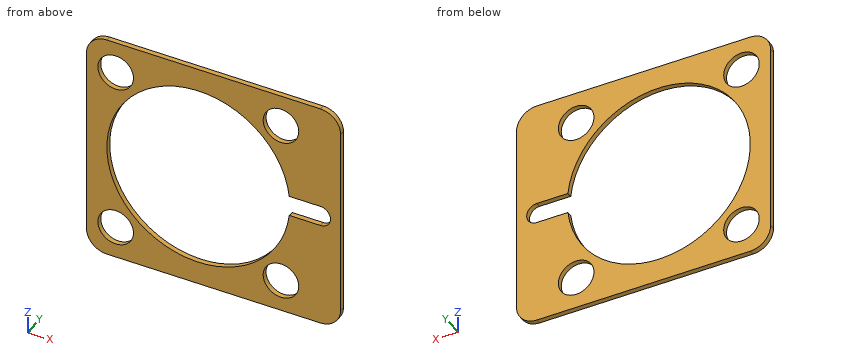
from build123d import *

# Parameters (mm, degrees)
SKETCH1_R           = 3.5
BOSS_EXTRUDE1_DEPTH = 1


with BuildPart() as part:
    # Sketch1 → Boss-Extrude1 (new body)
    with BuildSketch(Plane(origin=(0, 0, 0), x_dir=(1, 0, 0), z_dir=(0, 1, 0))):
        with BuildLine():
            Line((-21, -22.5), (21, -22.5))
            ThreePointArc((21, -22.5), (23.828427125, -21.328427125), (25, -18.5))
            Line((25, -18.5), (25, 18.5))
            ThreePointArc((25, 18.5), (23.828427125, 21.328427125), (21, 22.5))
            Line((21, 22.5), (-21, 22.5))
            ThreePointArc((-21, 22.5), (-23.828427125, 21.328427125), (-25, 18.5))
            Line((-25, 18.5), (-25, -18.5))
            ThreePointArc((-25, -18.5), (-23.828427125, -21.328427125), (-21, -22.5))
        make_face()
        with Locations((-19.263455967, 16.263455967)):
            Circle(SKETCH1_R, mode=Mode.SUBTRACT)
        with Locations((13.263455967, 16.263455967)):
            Circle(SKETCH1_R, mode=Mode.SUBTRACT)
        with Locations((13.263455967, -16.263455967)):
            Circle(SKETCH1_R, mode=Mode.SUBTRACT)
        with Locations((-19.263455967, -16.263455967)):
            Circle(SKETCH1_R, mode=Mode.SUBTRACT)
        with BuildLine():
            Line((15, 2), (21, 2))
            ThreePointArc((21, 2), (23, 0), (21, -2))
            Line((21, -2), (15, -2))
            ThreePointArc((15, -2), (14.944422982, -1.99922765), (14.888888889, -1.996911195))
            ThreePointArc((14.888888889, -1.996911195), (-21, 0), (14.888888889, 1.996911195))
            ThreePointArc((14.888888889, 1.996911195), (14.944422982, 1.99922765), (15, 2))
        make_face(mode=Mode.SUBTRACT)
    extrude(amount=BOSS_EXTRUDE1_DEPTH)


solid = part.part
Can you work these out from the model? Positions are in its coordinate system, mm. Coordinates: 2 decimals unless noted, no trailing zeros. Write each loop counter-clockwise with the first axis right and the second up, starting at its lowest first coordinate (ties: lowest second). Pieces come first, ordered by that corner, then holes. Notation, with made-up numbers: (36.25, 39) -> (92.25, 39) arc R12 cw to (92.25, 47) -> close; hole circle Ø7 at (48, 77). An arc over 180 degrees is marked (long way). Write each question's results on one line, items separated by ' | '. Start each with the question number.
Q1. If I drill on probe 1 along Z at (x, y) = (15, 0.7); probe 2 along X at (y, z) = (0.8, 0); probe 3 along X at (y, z) = (0.6, -14), over which ranges is the centre line in solid material (lowest first)?
Q2. Imagine slicing it at D-D (y = 0.3). Write out the boundary of the cut face in (x, z), then the cut area to 3 significant figures.
Q3. I'm going to push a flat-ended pin straight in: pin 1 (4 mm diameter, centred on x = 13.26, z = -16.26, fed in from -Y). Where does the tip first touch, or does it pass through?
Q4. Imagine slicing it at B-B (x = -3). Write out the boundary of the cut face in (y, z), then the cut area to 3 significant figures.
Q5. Imagine slicing it at A-A (z = 0). Write out the boundary of the cut face in (x, y), then the cut area to 3 significant figures.
Q6. Imagine slicing it at C-C (z = -15). Write out the boundary of the cut face in (x, y), then the cut area to 3 significant figures.
Taken from the geometry:
1) probe 1: z = -22.5 to -19.3, -13.22 to -2, 2 to 13.22, 19.3 to 22.5 | probe 2: x = -25 to -21, 23 to 25 | probe 3: x = -25 to -21.93, -16.59 to -14.31, 8.31 to 10.59, 15.93 to 25
2) outline: (-25, -18.5) arc R4 ccw to (-21, -22.5) -> (21, -22.5) arc R4 ccw to (25, -18.5) -> (25, 18.5) arc R4 ccw to (21, 22.5) -> (-21, 22.5) arc R4 ccw to (-25, 18.5) -> close; hole circle Ø7 at (-19.26, -16.26); hole circle Ø7 at (-19.26, 16.26); hole circle Ø7 at (13.26, -16.26); hole circle Ø7 at (13.26, 16.26); hole (14.89, -2) arc R2 ccw to (15, -2) -> (21, -2) arc R2 ccw to (21, 2) -> (15, 2) arc R2 ccw to (14.89, 2) arc R18 ccw (long way) to start | area: 1,030 mm^2
3) pin 1: passes through
4) outline: (0, -22.5) -> (1, -22.5) -> (1, -18) -> (0, -18) -> close; (0, 18) -> (1, 18) -> (1, 22.5) -> (0, 22.5) -> close | area: 9.00 mm^2
5) outline: (-25, 0) -> (-21, 0) -> (-21, 1) -> (-25, 1) -> close; (23, 0) -> (25, 0) -> (25, 1) -> (23, 1) -> close | area: 6.00 mm^2
6) outline: (-25, 0) -> (-22.53, 0) -> (-22.53, 1) -> (-25, 1) -> close; (-16, 0) -> (-12.95, 0) -> (-12.95, 1) -> (-16, 1) -> close; (6.95, 0) -> (10, 0) -> (10, 1) -> (6.95, 1) -> close; (16.53, 0) -> (25, 0) -> (25, 1) -> (16.53, 1) -> close | area: 17.0 mm^2
